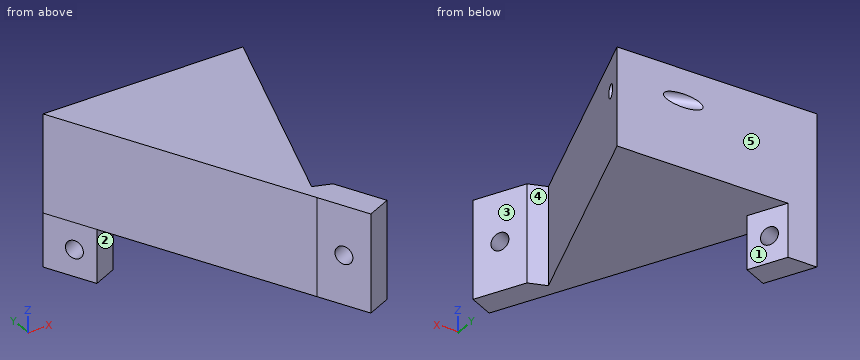
```python
from build123d import *

# Parameters (mm, degrees)
BOSS_EXTRUDE1_DEPTH = 22
SKETCH6_W           = 12
SKETCH6_H           = 12
SKETCH6_W_2         = 22
BOSS_EXTRUDE4_DEPTH = 6
BOSS_EXTRUDE5_DEPTH = 22
SKETCH9_R           = 2
CUT_EXTRUDE9_DEPTH  = 6
SKETCH10_R          = 1.5
CUT_EXTRUDE10_DEPTH = 36
CUT_EXTRUDE11_DEPTH = 36


with BuildPart() as part:
    # Sketch1 → Boss-Extrude1 (new body)
    with BuildSketch(Plane.XY):
        Polygon((-36.238637744, 24.241346543), (-9.742760301, -30.758653457), (9.494123696, 24.241346543), align=None)
    extrude(amount=BOSS_EXTRUDE1_DEPTH)

    # Sketch6 → Boss-Extrude4 (add)
    with BuildSketch(Plane(origin=(-19.934259386, -9.603194429, 0), x_dir=(0, 0, 1), z_dir=(-0.9009094793526655, -0.4340070391278342, 0))):
        with Locations((-6, 31.567082762)):
            Rectangle(SKETCH6_W, SKETCH6_H)
        with Locations((11, -29.48233592)):
            Rectangle(SKETCH6_W_2, SKETCH6_H)
    extrude(amount=-BOSS_EXTRUDE4_DEPTH)


with BuildPart() as boss_extrude4_piece_1:
    # of the separate pieces the step leaves, piece 1, a body of its own (boss_extrude4_pieces)
    add(part.part.solids().sort_by_distance((-36.238637744, 24.241346543, 0))[0])



with BuildPart() as boss_extrude4_piece_2:
    # of the separate pieces the step leaves, piece 2, a body of its own (boss_extrude4_pieces)
    add(part.part.solids().sort_by_distance((-4.337303425, -28.154611222, 0))[0])


with BuildPart() as boss_extrude4_piece_1_1:
    add(boss_extrude4_piece_1.part)

    add(boss_extrude4_piece_2.part)  # Boss-Extrude5 merges Boss-Extrude4 piece 2
    # Sketch8 → Boss-Extrude5 (add)
    with BuildSketch(Plane(origin=(0, 0, 0), x_dir=(-1, 0, 0), z_dir=(0, 0, -1))):
        Polygon((9.742760301, -30.758653457), (4.337303425, -28.154611222), (8.343083331, -26.756849768), align=None)
    extrude(amount=-BOSS_EXTRUDE5_DEPTH)

    # Sketch9 → Cut-Extrude9 (cut)
    with BuildSketch(Plane(origin=(-14.52880251, -6.999152194, 0), x_dir=(0, 0, -1), z_dir=(0.9009094793526653, 0.43400703912783434, 0))):
        with Locations(Location((6, 30.567082762, 0), (0, 0, 90))):
            Circle(SKETCH9_R)
        with Locations(Location((-11, -29.48233592, 0), (0, 0, 90))):
            Circle(SKETCH9_R)
    extrude(amount=-CUT_EXTRUDE9_DEPTH, mode=Mode.SUBTRACT)

    # Sketch10 → Cut-Extrude10 (cut)
    with BuildSketch(Plane(origin=(0.904752149, -0.316447493, 0), x_dir=(0, 0, -1), z_dir=(0.9439285225355003, -0.3301498816355197, 0))):
        with Locations(Location((-15, 21.016582241, 0), (0, 0, 90))):
            Circle(SKETCH10_R)
    extrude(amount=-CUT_EXTRUDE10_DEPTH, mode=Mode.SUBTRACT)

    # Sketch11 → Cut-Extrude11 (cut)
    with BuildSketch(Plane.XY):
        Polygon((-36.238637744, 24.241346543), (-29.578701161, 24.241346543), (-30.833180868, 26.845388778), align=None)
    extrude(amount=-CUT_EXTRUDE11_DEPTH, mode=Mode.SUBTRACT)


solid = boss_extrude4_piece_1_1.part
```
Build history of the part. All positions in model axes, mm. Face numbers are marked on the shaded views. A direction names the side the tool comes from. Give positions to 0.01 mm unless a question says otherwise; leave off trailing zeros. Loops run counter-clockwise (first coordinate to the right, second up) from the corner with the lowest first, then second, coordinate; pieces in that order, holes last.
Item 1: Slice it at C-C, the plane y = -6. List the corners of the cut face in (x, z).
Answers follow:
outline: (-21.67, 0) - (-1.08, 0) - (-1.08, 22) - (-21.67, 22) - close
Item 2: Which spindle directions (+Z, -Z, +X, -X, +Y, -Y) get a long thin tool onto all of the face, cutting with end or side? Do the marked faces 4 and 5. Say none if no direction does.
Answers follow:
face 4: +Z, -Z, +X
face 5: +Z, -Z, +X, -X, +Y
Item 3: Pull direction Y, two halves, no side cores. Call the marked faces 1, 2 and 3: released by +Y, released by -Y, zero draft, split by the parting line, or undercut.
Answers follow:
face 1: released by +Y
face 2: released by -Y
face 3: undercut
Item 4: Slice it at D-D, the plane x = -11. List the corners of the cut face in (y, z), and give its area (3 significant figures).
Answers follow:
outline: (-28.15, 0) - (24.24, 0) - (24.24, 22) - (-28.15, 22) - close
area: 1,150 mm2
Item 5: Slice it at B-B, the plane x = -3.5. Give the number of separate pieces and of enclosed holes in the cut face, and give its area (3 significant figures).
Answers follow:
separate pieces: 2
enclosed holes: 1
area: 1,040 mm2
Item 6: Flat gauge pins, fed straight in: pin 1 (10 mm diameter, centred on x = -8.5, z = 1, fed in from -Y); pin 2 (12 mm diameter, centred on x = -1, y = -6.5, fed in from -Z); pin 3 (12 mm diameter, centred on x = -23.5, z = -8, fed in from +Y); pin 4 (2 mm diameter, centred on y = -24, z = 7, fed in from +X). Where does each tip first touch, or does it go through?
Answers follow:
pin 1: stops at y = -41.57
pin 2: stops at z = 0
pin 3: stops at y = 24.08
pin 4: stops at x = -7.03
Item 7: Slice it at A-A, the plane z = 6.5. List the corners of the cut face in (x, y), and give its area (3 significant figures).
Answers follow:
outline: (-36.24, 24.24) - (-4.53, -41.57) - (0.87, -38.97) - (-4.34, -28.15) - (-8.34, -26.76) - (9.49, 24.24) - close
area: 1,340 mm2
Item 8: Drill centre lines: line 1 (Z direction, x = -7.5, y = -6); line 2 (Y direction, x = -30, z = -5); line 3 (Y direction, x = -15.5, z = 9). Where is each one in solid material? Low to high.
Answers follow:
line 1: z = 0 to 22
line 2: y = 13.93 to 17.55, 21.4 to 24.24
line 3: y = -18.81 to 24.24
